Autodesk Inventor part; units mm, degrees
ref_plane "YZ Plane" through (0, 0, 0) normal (1, 0, 0) x (0, 1, 0)
ref_plane "XZ Plane" through (0, 0, 0) normal (0, 1, 0) x (-1, 0, 0)
ref_plane "XY Plane" through (0, 0, 0) normal (0, 0, 1) x (1, 0, 0)
sketch "Sketch1" plane through (0, 0, 0) normal (0, 1, 0) x (-1, 0, 0)
  line L0 (0, -7.3152) -> (-6.3351, -3.6576)
  line L1 (-6.3351, -3.6576) -> (-6.3351, 3.6576)
  line L2 (-6.3351, 3.6576) -> (0, 7.3152)
  line L3 (0, 7.3152) -> (6.3351, 3.6576)
  line L4 (6.3351, 3.6576) -> (6.3351, -3.6576)
  line L5 (6.3351, -3.6576) -> (0, -7.3152)
  point P0 (0, 0)
  point P1 (0, 0)
  dimension "d0" = 7.3152
extrude "Extrusion1" add sketch "Sketch1" along normal blind 127
Build history of the part. All positions in model axes, mm. Round coordinates to 2 decimals unless told otherwise and drop trailing zeros. Write each loop counter-clockwise with the first axis right and the second up, starting at its lowest first coordinate (ties: lowest second). Pieces come first, ordered by that corner, then holes. Notation, with made-up numbers: (85.25, 44) -> (116.25, 44) arc R9 cw to (116.25, 51) -> close; hole circle Ø8 at (-33.75, -30.5). An arc over 180 degrees is marked (long way). Put each result on its own line as item: value.
Item 1: Slice it at C-C, the plane z = -6. Give the cut face in (x, y).
Here are the results:
outline: (-2.28, 0) -> (2.28, 0) -> (2.28, 127) -> (-2.28, 127) -> close
Item 2: Slice it at B-B, the plane x = 3.75. Give the cut face in (y, z), plus the area to 3 significant figures.
Here are the results:
outline: (0, -5.15) -> (127, -5.15) -> (127, 5.15) -> (0, 5.15) -> close
area: 1,310 mm^2
Item 3: Flat gauge pins, fed straight in: P1, Ø1.5, axis at x = -1, y = 20.5, coming from the +Z side; P2, Ø1, axis at x = 5, y = 47.5, coming from the +Z side; P3, Ø1, axis at x = 1, y = 71, coming from the +Z side. Where does each tip first touch, or does it go through?
Here are the results:
P1: stops at z = 7.17
P2: stops at z = 4.72
P3: stops at z = 7.03
Item 4: Wall check: probe 1 along X at (y, z) = (104.5, 6.75); probe 2 along Z at (x, y) = (-2.5, 9); probe 3 along X at (y, z) = (45.5, 4.25). Give the ranges that are in metal, low to high. Write a range as from..to.
Here are the results:
probe 1: x = -0.98..0.98
probe 2: z = -5.87..5.87
probe 3: x = -5.31..5.31
Item 5: Slice it at A-A, the plane y = 43. Give the cut face in (x, z).
Here are the results:
outline: (-6.34, -3.66) -> (0, -7.32) -> (6.34, -3.66) -> (6.34, 3.66) -> (0, 7.32) -> (-6.34, 3.66) -> close
